Autodesk Inventor part; units mm, degrees
ref_plane "YZ Plane" through (0, 0, 0) normal (1, 0, 0) x (0, 1, 0)
ref_plane "XZ Plane" through (0, 0, 0) normal (0, 1, 0) x (-1, 0, 0)
ref_plane "XY Plane" through (0, 0, 0) normal (0, 0, 1) x (1, 0, 0)
sketch "Sketch1" plane through (0, 0, 0) normal (0, 0, 1) x (1, 0, 0)
  line L0 (0, 0) -> (100, 0)
  line L1 (100, 0) -> (100, 100)
  line L2 (100, 100) -> (0, 100)
  line L3 (0, 100) -> (0, 0)
  dimension "d0" = 100
  dimension "d1" = 100
extrude "Extrusion1" add sketch "Sketch1" along normal blind 80
sketch "Sketch2" plane through (0, 0, 80) normal (0, 0, 1) x (1, 0, 0)
  line L0 (0, 100) -> (0, 0)
  line L1 (0, 50) -> (10, 50)
  line L2 (100, 100) -> (0, 100)
  line L3 (50, 100) -> (50, 75)
  line L4 (100, 0) -> (100, 100)
  line L5 (100, 53.1095) -> (100, 43.1095)
  line L6 (100, 43.1095) -> (90, 43.1095)
  line L7 (0, 0) -> (100, 0)
  line L8 (10, 75) -> (90, 75)
  line L9 (90, 75) -> (90, 0)
  line L10 (90, 0) -> (10, 0)
  line L11 (10, 0) -> (10, 75)
  dimension "d4" = 10
  dimension "d5" = 25
  dimension "d6" = 10
  dimension "d7" = 10
extrude "Extrusion2" cut sketch "Sketch2" against normal blind 80 contours L11 L8 L9 L7
sketch "Sketch3" plane through (0, 100, 0) normal (0, 1, 0) x (1, 0, 0)
  line L0 (90, 0) -> (10, 0)
  line L1 (32.4733, 0) -> (52.4733, 0)
  line L2 (52.4733, 0) -> (52.4733, -20)
  line L3 (10, -80) -> (90, -80)
  line L4 (70.0717, -80) -> (50.0717, -80)
  line L5 (50.0717, -80) -> (50.0717, -60)
  point P0 (0, 0)
  dimension "d10" = 20
  dimension "d11" = 20
  dimension "d12" = 20
  dimension "d13" = 20
sketch "Sketch4" plane through (0, 100, 0) normal (0, 1, 0) x (1, 0, 0)
  line L0 (0, 0) -> (0, -80)
  line L1 (0, -49.1237) -> (0, -24.1237)
  line L2 (0, -24.1237) -> (25, -24.1237)
  line L3 (100, 0) -> (100, -80)
  line L4 (100, -53.0628) -> (100, -28.0628)
  line L5 (100, -28.0628) -> (75, -28.0628)
  line L6 (25, -20.093) -> (75, -20.093)
  line L7 (75, -20.093) -> (75, -30.093)
  line L8 (75, -30.093) -> (25, -30.093)
  line L9 (25, -30.093) -> (25, -20.093)
  line L10 (33.3829, -30.093) -> (33.3829, -30.0462)
  line L11 (33.3829, -30.0462) -> (53.3829, -30.0462)
  line L12 (53.3829, -30.0462) -> (53.3829, -50.0462)
  line L13 (25, -50.0462) -> (75, -50.0462)
  line L14 (75, -50.0462) -> (75, -60.0462)
  line L15 (75, -60.0462) -> (25, -60.0462)
  line L16 (25, -60.0462) -> (25, -50.0462)
  point P0 (53.3829, -30.093)
  dimension "d14" = 25
  dimension "d15" = 25
  dimension "d16" = 90
  dimension "d18" = 25
  dimension "d19" = 90
  dimension "d20" = 50
  dimension "d21" = 10
  dimension "d22" = 20
  dimension "d23" = 20
  dimension "d24" = 50
  dimension "d25" = 10
extrude "Extrusion3" add sketch "Sketch4" along normal blind 200 contours L13 L14 L15 L16 | L6 L7 L8 L12 L11 L10 L9
sketch "Sketch5" plane through (75, 100, 20.093) normal (0, 0, -1) x (-1, 0, 0)
  point P0 (75, -100)
sketch "Sketch6" plane through (75, 100, 20.093) normal (0, 0, -1) x (-1, 0, 0)
  line L0 (0, 0) -> (0, 200)
  line L1 (0, 200) -> (25, 200)
  line L2 (21.6171, 200) -> (0, 200)
  line L3 (25, 200) -> (25, 165)
  circle A0 centre (25, 165) radius 2.5
  point P0 (75, -100)
  dimension "d28" = 25
  dimension "d29" = 35
  dimension "d30" = 5
extrude "Extrusion4" cut sketch "Sketch6" against normal blind 200
sketch "Sketch7" plane through (100, 0, 0) normal (1, 0, 0) x (0, 0, -1)
  line L0 (0, 0) -> (-80, 0)
  line L1 (-40, 0) -> (-40, 14)
  line L2 (-40, 0) -> (-40, 29.8709)
  line L3 (-39.9627, -1.129) -> (-39.9627, 29.871)
  circle A0 centre (-39.9627, 29.871) radius 15.8
  dimension "d33" = 14
  dimension "d34" = 31
  dimension "d35" = 31
  dimension "d36" = 31.6
extrude "Extrusion5" cut sketch "Sketch7" against normal blind 200 contours A0
properties part number "S.Platform"
CAD build for the part. Positions are in the model's coordinates, mm. A direction names the side the tool comes from. Round coordinates to 2 decimals unless told otherwise and drop trailing zeros. Loops run counter-clockwise (first coordinate to the right, second up) from the corner with the lowest first, then second, coordinate; pieces in that order, holes last.
(1) Drop flat-ended pins along their axis: pin 1 (8 mm diameter, centred on x = 32, y = 176, fed in from +Z); pin 2 (4 mm diameter, centred on x = 52, z = 27.5, fed in from -Y); pin 3 (5 mm diameter, centred on y = 242.5, z = 55.5, fed in from -X); pin 4 (4 mm diameter, centred on x = 50, y = 265, fed in from +Z). Give the stop position or say it passes through.
(2) Cut at D-D (z = 67.5). Give the cut face in (x, y).
(3) Cut at A-A (z = 53). Give the cut face in (x, y), plus the area to 3 significant figures.
(4) Wall check: line 1 along Y through (x, z) = (50, 52); line 2 along Z through (x, y) = (32, 232); line 3 along X through (y, z) = (45, 19). Give the ranges that are in metal, low to high.
(5) Two-plate mould, pull along X, no slides. Class faces 1 (the flat face through (25, 199, 25)), 2 (the flat face through (10, 45, 32)), 3 (the flat face through (50, 199, 60.046)): +X half, -X half, draft (parallel to the pull), parting line (faces both ways), or undercut.
(6) Cut at C-C (x = 65.5). Give the cut face in (y, z).
(7) Which spindle directions (+Z, -Z, +X, -X, +Y, -Y) get a long thin tool onto all of the face, cutting with end or side? Do faces 4 (the flat face through (64, 199, 30.093)), 5 (the flat face through (25, 199, 55)), 6 (the flat face through (75, 199, 25)). Say none if no direction does.
(8) Cut at B-B (y = 61.5). Give the cut face in (x, z), plus the area to 3 significant figures.
Findings below:
1. pin 1: stops at z = 60.05
1. pin 2: stops at y = 75
1. pin 3: stops at x = 25
1. pin 4: passes through
2. outline: (0, 0) - (10, 0) - (10, 75) - (90, 75) - (90, 0) - (100, 0) - (100, 100) - (0, 100) - close
3. outline: (0, 0) - (10, 0) - (10, 20.95) - (0, 20.95) - close; (0, 38.8) - (10, 38.8) - (10, 75) - (90, 75) - (90, 38.8) - (100, 38.8) - (100, 100) - (75, 100) - (75, 300) - (25, 300) - (25, 100) - (0, 100) - close; (90, 0) - (100, 0) - (100, 20.95) - (90, 20.95) - close; hole circle Ø5 at (50, 265)
3. area: 13,600 mm2
4. line 1: y = 75 to 262.5, 267.5 to 300
4. line 2: z = 20.09 to 30.09, 50.05 to 60.05
4. line 3: x = 0 to 10, 90 to 100
5. face 1: -X half
5. face 2: undercut
5. face 3: draft
6. outline: (75, 0) - (100, 0) - (100, 20.09) - (300, 20.09) - (300, 30.09) - (100, 30.09) - (100, 50.05) - (300, 50.05) - (300, 60.05) - (100, 60.05) - (100, 80) - (75, 80) - close
7. face 4: +X, -X, +Y
7. face 5: +Z, -Z, -X, +Y
7. face 6: +Z, -Z, +X, +Y
8. outline: (0, 0) - (10, 0) - (10, 80) - (0, 80) - close; (90, 0) - (100, 0) - (100, 80) - (90, 80) - close
8. area: 1,600 mm2
